from build123d import *

# Parameters (mm, degrees)
SALIENTE_EXTRUIR1_DEPTH = 15
CROQUIS3_R              = 14.29
CORTAR_EXTRUIR2_DEPTH   = 499.221807184
SALIENTE_EXTRUIR2_DEPTH = 15
SALIENTE_EXTRUIR3_DEPTH = 15
CROQUIS6_R              = 14.29
SALIENTE_EXTRUIR4_DEPTH = 15


with BuildPart() as part:
    # Croquis1 → Saliente-Extruir1 (new body)
    with BuildSketch(Plane(origin=(0, 0, 0), x_dir=(1, 0, 0), z_dir=(0, 1, 0))):
        with BuildLine():
            Line((28.62028588, 380.086840422), (-203.253807163, -15.179678662))
            ThreePointArc((-203.253807163, -15.179678662), (-244.309678662, -25.876192837), (-255.006192837, 15.179678662))
            Line((-255.006192837, 15.179678662), (-23.132099794, 410.446197745))
            ThreePointArc((-23.132099794, 410.446197745), (17.923771705, 421.142711921), (28.62028588, 380.086840422))
        make_face()
    extrude(amount=SALIENTE_EXTRUIR1_DEPTH)

    # Croquis3 → Cortar-Extruir2 (cut, through all)
    with BuildSketch(Plane(origin=(0, 15, 0), x_dir=(1, 0, 0), z_dir=(0, 1, 0))):
        with Locations(Location((-229.13, 0, 0), (0, 0, 270))):
            Circle(CROQUIS3_R)
        with Locations(Location((2.744093043, 395.266519084, 0), (0, 0, 270))):
            Circle(CROQUIS3_R)
    extrude(amount=-CORTAR_EXTRUIR2_DEPTH, mode=Mode.SUBTRACT)

    # Croquis4 → Saliente-Extruir2 (add, through all)
    with BuildSketch(Plane(origin=(0, 15, 0), x_dir=(1, 0, 0), z_dir=(0, 1, 0))):
        Polygon((-113.288910537, 95.628521871), (-129.646022382, 110.296576517), (-77.815690841, 198.649675659), (-46.271672707, 170.362934935), align=None)
    extrude(amount=-SALIENTE_EXTRUIR2_DEPTH)

    # Croquis5 → Saliente-Extruir3 (add, through all)
    with BuildSketch(Plane(origin=(0, 15, 0), x_dir=(1, 0, 0), z_dir=(0, 1, 0))):
        with BuildLine():
            Line((155.952842447, 395.874026356), (88.935604616, 321.139613292))
            ThreePointArc((88.935604616, 321.139613292), (53.823388605, 345.447170601), (11.459302657, 350.833196717))
            Line((11.459302657, 350.833196717), (21.614505852, 387.987304257))
            Line((21.614505852, 387.987304257), (17.093708134, 410.446197745))
            Line((17.093708134, 410.446197745), (-23.132099794, 410.446197745))
            ThreePointArc((-23.132099794, 410.446197745), (-16.015624614, 418.677477916), (-6.431242037, 423.828963415))
            ThreePointArc((-6.431242037, 423.828963415), (80.317160754, 442.127171951), (155.952842447, 395.874026356))
        make_face()
    extrude(amount=-SALIENTE_EXTRUIR3_DEPTH)

    # Croquis6 → Saliente-Extruir4 (add)
    with BuildSketch(Plane(origin=(0, 0, 0), x_dir=(-1, 0, 0), z_dir=(0, -1, 0))):
        with BuildLine():
            Line((16.370108222, 303.393509849), (-7.031750258, 366.185372475))
            Line((-7.031750258, 366.185372475), (-88.935604616, 345.894949454))
            Line((-88.935604616, 345.894949454), (-88.935604616, 321.139613292))
            ThreePointArc((-88.935604616, 321.139613292), (-94.698962335, 313.085487939), (-101.541302009, 305.925347215))
            ThreePointArc((-101.541302009, 305.925347215), (-108.68476793, 255.708040538), (-58.018177093, 253.319826096))
            ThreePointArc((-58.018177093, 253.319826096), (-17.827653511, 273.905315038), (16.370108222, 303.393509849))
        make_face()
        with Locations(Location((-82.26486862, 277.566517623, 0), (0, 0, 90))):
            Circle(CROQUIS6_R, mode=Mode.SUBTRACT)
    extrude(amount=-SALIENTE_EXTRUIR4_DEPTH)


solid = part.part
For this review, take the finished solid that the model builds, in its own axes (mm). A direction names the side the tool comes from. Round coordinates to 2 decimals unless told otherwise and drop trailing zeros. Write each loop counter-clockwise with the first axis right and the second up, starting at its lowest first coordinate (ties: lowest second). Pieces come first, ordered by that corner, then holes. Notation, with made-up numbers: (87.25, 12.5) - (133.25, 12.5) arc R20 cw to (133.25, 48.5) - close; hole circle Ø2 at (8.25, -2). An arc over 180 degrees is marked (long way). Write item = value, one per line. Start each with the question number.
1. Consider section A-A on z = 0. State the section outline as (x, y) points.
2. Consider section B-B on x = -229.13. State the section outline as (y, z) points, plus the area to 3 significant figures.
3. Consider section D-D on z = -65.5. State the section outline as (x, y) points, plus the area to 3 significant figures.
4. For faces 1 (the face through (-121.4, 7.6, -102.9)), 2 (the face through (79.063, 7.605, -442.336)), 3 (the face through (94.61, 7.4, -313.19)), list the 3-axis set-ups (+Z, -Z, +X, -X, +Y, -Y) from which the entire face can be reached by the end or side of a thin tool; tool diameter is ignored.
5. Draft analysis for pull direction X (two halves, no side actions). For faces 4 (the face through (-243.74, 7.4, 26.2)), 5 (the face through (-62.26, 7.6, -184.7)), 6 (the face through (-46.663, 7.395, -251.755)), state which applies: released by +X, released by -X, zero draft, split by the parting line, or undercut.
6. For pin 1 Ø17 at (x, z) = (-229.13, 0) entering from -Y; pin 2 Ø5 at (y, z) = (5, -369.5) entering from +X; pin 3 Ø6 at (y, z) = (11, -277) entering from -X; pin 4 Ø1.5 at (x, y) = (-3, 5.5) entering from -Z, all flat-tipped, find the tip position at first contact; note any pin that passes through.
7. Consider section C-C on y = 6. State the section outline as (x, z) points.
8. Wall thickness on L1, parallel to Z at x = -202.5, y = 9.5; L2, parallel to X at y = 9.75, z = -151; L3, parallel to X at y = 13.75, z = -8: over which ranges is each line inside the solid? List them lowest first.
Evaluation:
q1.outline = (-259.13, 0) - (-243.42, 0) - (-243.42, 15) - (-259.13, 15) - close; (-214.84, 0) - (-194.35, 0) - (-194.35, 15) - (-214.84, 15) - close
q2.outline = (0, -59.29) - (15, -59.29) - (15, -14.29) - (0, -14.29) - close; (0, 14.29) - (15, 14.29) - (15, 30) - (0, 30) - close
q2.area = 911 mm2
q3.outline = (-225.49, 0) - (-155.92, 0) - (-155.92, 15) - (-225.49, 15) - close
q3.area = 1,040 mm2
q4.face_1 = +Z, +Y, -Y
q4.face_2 = -Z, +Y, -Y
q4.face_3 = +X, +Y, -Y
q5.face_4 = split by the parting line
q5.face_5 = released by +X
q5.face_6 = undercut
q6.pin_1 = through
q6.pin_2 = 134.54
q6.pin_3 = -103.18
q6.pin_4 = -426.48
q7.outline = (-255.01, -15.18) - (-23.13, -410.45) arc R30 ccw to (-6.43, -423.83) arc R120 ccw to (155.95, -395.87) - (88.94, -321.14) arc R70 cw to (101.54, -305.93) arc R34.29 ccw (long way) to (58.02, -253.32) arc R190 ccw to (-16.37, -303.39) - (-77.82, -198.65) - (-46.27, -170.36) - (-113.29, -95.63) - (-129.65, -110.3) - (-203.25, 15.18) arc R30 ccw to start; hole circle Ø28.58 at (-229.13, 0); hole circle Ø28.58 at (2.74, -395.27); hole circle Ø28.58 at (82.26, -277.57)
q8.L1 = -104.68 to 13.89
q8.L2 = -175.33 to -63.64
q8.L3 = -258.04 to -240.97, -217.29 to -189.66
